Study the drawing (mm; zero at the part's minimum x, y, z) and answer. Give positions to 0.01 mm unless a question says otherwise; leave off trailing zeros. Order: outer loops, then holes, each group sorted by start corner. A loop starts at its lowest first (then second) coordinate and runs counter-clockwise, first axis right, second up. Notation, with made-up numbers: (36, 39) - (62, 39) arc R25 cw to (62, 77) - close; hole circle Ø1 at (-24.75, 37). An arc over 180 degrees is marked (long way). Return JSON: item names as keys, results as strings.
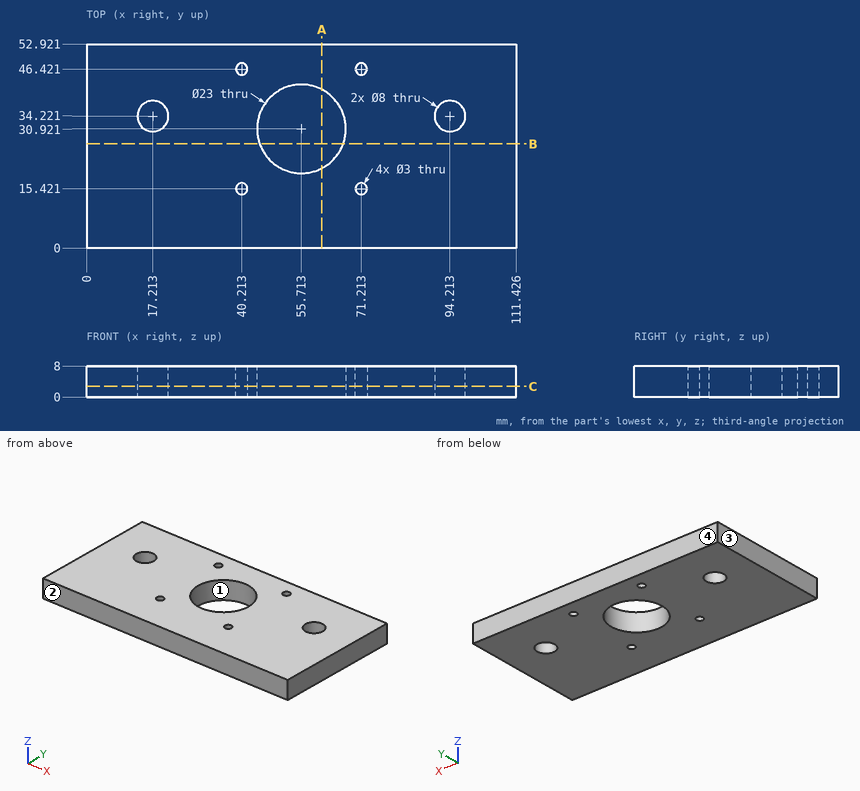
Q1. Determine the mould class of the marked faces 1, 2, 3 and 4 for opening direction Y: released by +Y, released by -Y, zero draft, split by the parting line, or undercut.
Values:
{"face 1": "undercut", "face 2": "released by -Y", "face 3": "zero draft", "face 4": "released by +Y"}
Q2. A cutting plane is placed at B-B (y = 27). Write down the section's boundary in (x, z).
Values:
{"outline": "(0, 0) - (44.9, 0) - (44.9, 8) - (0, 8) - close; (66.52, 0) - (111.43, 0) - (111.43, 8) - (66.52, 8) - close"}
Q3. Consider L1, parallel to X at y = 46.5, z = 4.5 (1 decimal); L2, parallel to X at y = 31, z = 4 (1 decimal); L3, parallel to X at y = 35, z = 4 (1 decimal). Determine where each line is inside the solid, lowest interval first.
Values:
{"L1": "x = 0 to 38.7, 41.7 to 69.7, 72.7 to 111.4", "L2": "x = 0 to 14.8, 19.6 to 44.2, 67.2 to 91.8, 96.6 to 111.4", "L3": "x = 0 to 13.3, 21.1 to 45, 66.5 to 90.3, 98.1 to 111.4"}
Q4. Given pin 1 (2.5 mm diameter, centred on x = 71.21, y = 46.42, fed in from -Z); pin 2 (2 mm diameter, centred on x = 65.5, z = 5, fed in from -Y), each flat-ended and moving along its own axis, determine where each tip first touches the part or whether it passes through.
Values:
{"pin 1": "passes through", "pin 2": "stops at y = 0"}
Q5. A cutting plane is placed at A-A (x = 61). Write down the section's boundary in (y, z).
Values:
{"outline": "(0, 0) - (20.71, 0) - (20.71, 8) - (0, 8) - close; (41.13, 0) - (52.92, 0) - (52.92, 8) - (41.13, 8) - close"}
Q6. A cutting plane is placed at C-C (z = 2.75). Write down the section's boundary in (x, y), and give its area (3 significant figures).
Values:
{"outline": "(0, 0) - (111.43, 0) - (111.43, 52.92) - (0, 52.92) - close; hole circle Ø8 at (17.21, 34.22); hole circle Ø3 at (40.21, 15.42); hole circle Ø3 at (40.21, 46.42); hole circle Ø23 at (55.71, 30.92); hole circle Ø3 at (71.21, 15.42); hole circle Ø3 at (71.21, 46.42); hole circle Ø8 at (94.21, 34.22)", "area": "5,350 mm²"}
